Work out the finished part from the listing and answer in its coordinate system (mm). A direction names the side the tool comes from. Round coordinates to 2 decimals unless told otherwise and drop trailing zeros. Order: outer loops, then holes, each group sorted by start corner. A loop starts at its lowest first (then second) coordinate and runs counter-clockwise, first axis right, second up. Notation, with made-up numbers: (78, 24) - (86, 24) arc R26 ccw to (86, 58) - close; hole circle Ø9 at (-13.5, -21.75). An arc over 180 degrees is marked (long way). Use CSV: the item, a comma, the result in double quotes.
from build123d import *

# Parameters (mm, degrees)
F1_DEPTH      = 6.35
F2_ANGLE_BACK = 22.5
F2_ANGLE      = 45
F4_DEPTH      = 25.401
F5_DEPTH      = 2.54


with BuildPart() as f1:
    # F0 (on Front) → F1 (new body, symmetric)
    with BuildSketch(Plane.XZ):
        Polygon((-9.525, 22.1488), (-9.525, 25.4), (-15.875, 25.4), (-15.875, 22.1488), (-19.05, 12.6238), (-6.35, 12.6238), align=None)
    extrude(amount=F1_DEPTH, both=True)

    # F0 (on Front) → F2 (revolve)
    with BuildSketch(Plane.XZ, mode=Mode.PRIVATE) as f2_sk:
        Polygon((-9.525, 25.4), (0, 25.4), (0, 39.37), (-25.4, 37.465), (-25.4, 25.4), (-15.875, 25.4), align=None)
    revolve(f2_sk.sketch.rotate(Axis((-30.5623934027, 0, 0), (-1, 0, 0)), -F2_ANGLE_BACK), axis=Axis((-30.5623934027, 0, 0), (-1, 0, 0)), revolution_arc=F2_ANGLE)

    # F3 (on face) → F4 (cut, through all)
    with BuildSketch(Plane.YZ):
        with BuildLine():
            Line((11.3784447312, 25.4), (10.5210244843, 25.4))
            Line((10.5210244843, 25.4), (9.7201591821, 23.4665401258))
            ThreePointArc((9.7201591821, 23.4665401258), (4.9552941792, 24.9119461222), (0, 25.4))
            Line((0, 25.4), (0, 22.86))
            Line((0, 22.86), (11.3784447312, 22.86))
            Line((11.3784447312, 22.86), (11.3784447312, 25.4))
        make_face()
        with BuildLine():
            Line((9.7201591821, 23.4665401258), (10.5210244843, 25.4))
            Line((10.5210244843, 25.4), (0, 25.4))
            ThreePointArc((0, 25.4), (4.9552941792, 24.9119461222), (9.7201591821, 23.4665401258))
        make_face()
        with BuildLine():
            Line((0, 22.86), (0, 25.4))
            ThreePointArc((0, 25.4), (-4.9552941792, 24.9119461222), (-9.7201591821, 23.4665401258))
            Line((-9.7201591821, 23.4665401258), (-10.5210244843, 25.4))
            Line((-10.5210244843, 25.4), (-11.5035856143, 25.4))
            Line((-11.5035856143, 25.4), (-11.5035856143, 22.86))
            Line((-11.5035856143, 22.86), (0, 22.86))
        make_face()
        with BuildLine():
            ThreePointArc((-9.7201591821, 23.4665401258), (-4.9552941792, 24.9119461222), (0, 25.4))
            Line((0, 25.4), (-10.5210244843, 25.4))
            Line((-10.5210244843, 25.4), (-9.7201591821, 23.4665401258))
        make_face()
    extrude(amount=-F4_DEPTH, mode=Mode.SUBTRACT)

    # F5 (add, through all): a face of the model
    f5_faces = [f1.faces().sort_by_distance(p)[0] for p in [
        (-12.7, 0, 22.86),
    ]]
    extrude(f5_faces, amount=F5_DEPTH)


solid = f1.part
(1) Find section D-D (x = -2.5). Determine the outline of the cut face in (y, z) (1 decimal), and give its area (3 significant figures).
Findings below:
outline,"(-15, 36.2) - (-10.5, 25.4) - (10.5, 25.4) - (15, 36.2) arc R39.2 ccw to start"
area,"336 mm²"
(2) The mould has two halves that part along Z. Classify faces 1 (the flat face through (-12.878, 12.825, 30.963)), 2 (the conical face through (-12.9, -0.2, 38.4)), 3 (the flat face through (-9.525, 0, 24)), 4 (the flat face through (-25.4, 2, 31)): released by +Z, released by -Z, zero draft, split by the parting line, or undercut.
Findings below:
face 1,"released by -Z"
face 2,"released by +Z"
face 3,"undercut"
face 4,"zero draft"
(3) For faces 5 (the flat face through (-13, 6.35, 18)), 6 (the flat face through (-13, -6.35, 18)), 7 (the flat face through (-7.915, -0.089, 17.32)), 8 (the flat face through (-17.44, -0.09, 17.45)), determine the directions among +Z, -Z, +X, -X, +Y, -Y from which every point of the face is accessible in a straight line to the end or side of a thin tool.
Findings below:
face 5,"-Z, +X, -X, +Y"
face 6,"-Z, +X, -X, -Y"
face 7,"+X, +Y, -Y"
face 8,"-X, +Y, -Y"
(4) Each of these flat-tipped pins is pushed along its axis until it touches: pin 1 (8 mm diameter, centred on x = -22, y = 5, fed in from +Z); pin 2 (2 mm diameter, centred on x = -2.5, y = -4, fed in from +Z); pin 3 (10 mm diameter, centred on x = -17, z = 27.5, fed in from -Y); pin 4 (3.5 mm diameter, centred on y = 1.5, z = 24, fed in from -X). Where does it stop, or does it pass through?
Findings below:
pin 1,"stops at z = 37.87"
pin 2,"stops at z = 39.1"
pin 3,"stops at y = -13.46"
pin 4,"stops at x = -25.4"
(5) Find the intervals of material crossed by L1, parallel to Z at x = -9.5, y = -9.5; L2, parallel to Y at x = -14.25, z = 20.25; L3, parallel to X at y = 1.5, z = 23.25 (3 decimals), in increasing order. Write a range as from..to.
Findings below:
L1,"z = 25.4..37.47"
L2,"y = -6.35..6.35"
L3,"x = -15.875..-9.525"
(6) Find section B-B (x = -9). Determine the outline of the cut face in (y, z) (3 decimals).
Findings below:
outline,"(-14.808, 35.75) - (-10.521, 25.4) - (10.521, 25.4) - (14.808, 35.75) arc R38.695 ccw to start; (-6.35, 12.624) - (6.35, 12.624) - (6.35, 20.574) - (-6.35, 20.574) - close"
(7) Find section C-C (z = 27.75). Determine the outline of the cut face in (x, y), and give its area (3 significant figures).
Findings below:
outline,"(-25.4, -11.49) - (0, -11.49) - (0, 11.49) - (-25.4, 11.49) - close"
area,"584 mm²"
